CAD build for the part. Positions are in the model's coordinates, mm. Face numbers are marked on the shaded views. Round coordinates to 2 decimals unless told otherwise and drop trailing zeros. Loops run counter-clockwise (first coordinate to the right, second up) from the corner with the lowest first, then second, coordinate; pieces in that order, holes last. Notation, with made-up numbers: (55.25, 25) -> (108.25, 25) arc R28 ccw to (108.25, 61) -> close; hole circle Ø11 at (13, 67.25). An arc over 180 degrees is marked (long way). Answer as CSV lines item,"result".
```python
from build123d import *

# Parameters (mm, degrees)
SKETCH1_R               = 11
SKETCH1_R_2             = 4
SKETCH1_R_3             = 1
BOSS_EXTRUDE1_DEPTH     = 5
SKETCH2_R               = 1.5
CUT_EXTRUDE1_DEPTH      = 10
CUT_EXTRUDE1_DEPTH_BACK = 10


with BuildPart() as part:
    # Sketch1 → Boss-Extrude1 (new body)
    with BuildSketch(Plane(origin=(0, 0, 0), x_dir=(1, 0, 0), z_dir=(0, 1, 0))):
        Circle(SKETCH1_R)
        Circle(SKETCH1_R_2, mode=Mode.SUBTRACT)
        with Locations((-8, 0)):
            Circle(SKETCH1_R_3, mode=Mode.SUBTRACT)
        with Locations((4, 6.92820323)):
            Circle(SKETCH1_R_3, mode=Mode.SUBTRACT)
        with Locations((4, -6.92820323)):
            Circle(SKETCH1_R_3, mode=Mode.SUBTRACT)
    extrude(amount=BOSS_EXTRUDE1_DEPTH)

    # Sketch2 → Cut-Extrude1 (cut, two sides)
    with BuildSketch(Plane(origin=(10.998674606, 0, 0), x_dir=(0, 0, -1), z_dir=(1, 0, 0))) as cut_extrude1_sk:
        with Locations((0.011578062, 2.49997319)):
            Circle(SKETCH2_R)
    extrude(amount=CUT_EXTRUDE1_DEPTH, mode=Mode.SUBTRACT)
    extrude(cut_extrude1_sk.sketch, amount=-CUT_EXTRUDE1_DEPTH_BACK, mode=Mode.SUBTRACT)


solid = part.part
```
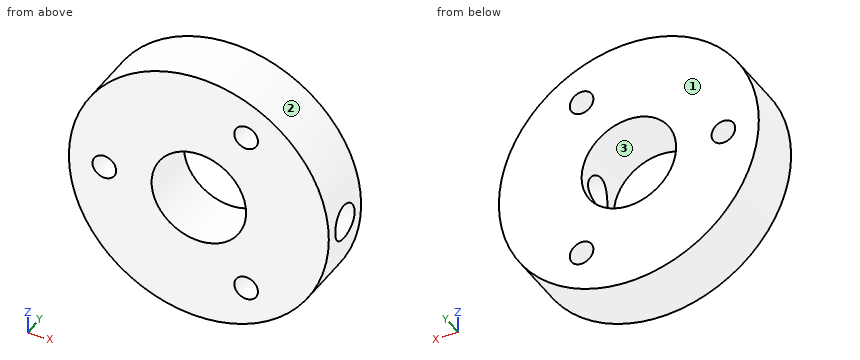
Q1. Probe L1, parallel to X at y = 2.25, z = 0; L2, parallel to Z at x = 0, y = 2.8; L3, parallel to Z at x = 4.75, y = 2.9. List the from-to ranges inside material, lowest first. Write a range as [from, to].
Results:
L1,"[-11, -9], [-7, -4]"
L2,"[-11, -4], [4, 11]"
L3,"[-9.92, -7.59], [-6.27, -1.46], [1.43, 6.27], [7.59, 9.92]"
Q2. Slice it at D-D, the plane z = -0.5. Give the cut face in (x, y).
Results:
outline,"(-10.99, 0) -> (-8.87, 0) -> (-8.87, 5) -> (-10.99, 5) -> close; (-7.13, 0) -> (-3.97, 0) -> (-3.97, 5) -> (-7.13, 5) -> close; (3.97, 0) -> (10.99, 0) -> (10.99, 1.08) -> (3.97, 1.08) -> close; (3.97, 3.92) -> (10.99, 3.92) -> (10.99, 5) -> (3.97, 5) -> close"
Q3. Two-plate mould, pull along Z, no slides. Class the marked faces 1, 2 and 3: pulls with the +Z half, pulls with the -Z half, needs draft (parallel to the pull), parting line crosses it, or undercut.
Results:
face 1,"needs draft"
face 2,"parting line crosses it"
face 3,"undercut"
Q4. Drop flat-ended pins along their axis: pin 1 Ø3 at (y, z) = (2, 2.5) entering from -X; pin 2 Ø7 at (x, z) = (0, 0) entering from +Y; pin 3 Ø1.5 at (y, z) = (3, 1.5) entering from +X. Give the stop position or say it passes through.
Results:
pin 1,"x = -10.95"
pin 2,"through"
pin 3,"x = 10.95"
Q5. Slice it at C-C, the plane y = 1.7. Give the cut face in (x, z).
Results:
outline,"(3.79, -1.28) arc R4 cw (long way) to (3.8, 1.26) -> (10.93, 1.26) arc R11 ccw (long way) to (10.93, -1.28) -> close; hole circle Ø2 at (-8, 0); hole circle Ø2 at (4, -6.93); hole circle Ø2 at (4, 6.93)"
Q6. Slice it at B-B, the plane z = 7.5. Give the cut face in (x, y).
Results:
outline,"(-8.05, 0) -> (3.18, 0) -> (3.18, 5) -> (-8.05, 5) -> close; (4.82, 0) -> (8.05, 0) -> (8.05, 5) -> (4.82, 5) -> close"
Q7. Slice it at A-A, the plane x = 0. Give the cut face in (y, z), and give its area (3 significant figures).
Results:
outline,"(0, -11) -> (5, -11) -> (5, -4) -> (0, -4) -> close; (0, 4) -> (5, 4) -> (5, 11) -> (0, 11) -> close"
area,"70.0 mm2"
